from build123d import *

# Parameters (mm, degrees)
EXTRUDE_1_DEPTH = 7.5


with BuildPart() as part:
    # 草图1 → 凸台-拉伸1 (new body, symmetric)
    with BuildSketch(Plane.XY):
        Polygon((1.356773133, 2.35), (-1.356773133, 2.35), (-2.713546265, 0), (-1.356773133, -2.35), (1.356773133, -2.35), (2.713546265, 0), align=None)
    extrude(amount=EXTRUDE_1_DEPTH, both=True)

    # 草图3 → Hole Wizard 387 (revolve, cut)
    with BuildSketch(Plane(origin=(0, 0, 7.5), x_dir=(0, -1, 0), z_dir=(1, 0, 0))):
        Polygon((0, 0), (0, 8.751075774), (1.25, 8), (1.25, 0), align=None)
    hole_wizard_387 = revolve(axis=Axis((0, 0, 13.85), (0, 0, -1)), mode=Mode.SUBTRACT)

    # 镜向1: Hole Wizard 387 across plane
    add(hole_wizard_387.mirror(Plane.XY), mode=Mode.SUBTRACT)


solid = part.part
Design review of the part built by this model. Coordinates are the model's own, in mm. Coordinates: 2 decimals unless noted, no trailing zeros. Write each loop counter-clockwise with the first axis right and the second up, starting at its lowest first coordinate (ties: lowest second). Pieces come first, ordered by that corner, then holes. Notation, with made-up numbers: (40, 85) - (65, 85) arc R12 cw to (65, 99) - close; hole circle Ø4 at (34, 48). An arc over 180 degrees is marked (long way). Use one line per item in the form item = value.
Q1. For probe 1 along Y at (x, z) = (0, -2.25); probe 2 along X at (y, z) = (-1, 5.5); probe 3 along X at (y, z) = (0.5, -4.25), list the stretches that pass through material, from the lowest coordinate up.
Taken from the geometry:
probe_1 = -2.35 to -1.25, 1.25 to 2.35
probe_2 = -2.14 to -0.75, 0.75 to 2.14
probe_3 = -2.42 to -1.15, 1.15 to 2.42
Q2. Consider section D-D (y = 2). Write out the cut boundary in (x, z).
Taken from the geometry:
outline = (-1.56, -7.5) - (1.56, -7.5) - (1.56, 7.5) - (-1.56, 7.5) - close
Q3. Consider section C-C (y = 0.9). Write out the cut boundary in (x, z), plus the area to 3 significant figures.
Taken from the geometry:
outline = (-2.19, -7.5) - (-0.87, -7.5) - (-0.87, 7.5) - (-2.19, 7.5) - close; (0.87, -7.5) - (2.19, -7.5) - (2.19, 7.5) - (0.87, 7.5) - close
area = 39.8 mm^2
Q4. Consider section A-A (x = 0). Write out the cut boundary in (y, z), plus the area to 3 significant figures.
Taken from the geometry:
outline = (-2.35, -7.5) - (-1.25, -7.5) - (-1.25, 7.5) - (-2.35, 7.5) - close; (1.25, -7.5) - (2.35, -7.5) - (2.35, 7.5) - (1.25, 7.5) - close
area = 33.0 mm^2
Q5. The part is to be moulded in two halves that separate along Y. For faces 1 (the flat face through (1, 1, 7.5)), 2 (the cylindrical face through (1.22, 0.27, -0.11)), 3 (the flat face through (-2.045, -1.159, 0.105)), 4 (the flat face through (0, 2.35, 0)), say which applies: +Y half, -Y half, draft (parallel to the pull), parting line (faces both ways), or undercut.
Taken from the geometry:
face_1 = draft
face_2 = undercut
face_3 = -Y half
face_4 = +Y half
Q6. Consider section B-B (z = 4.5). Write out the cut boundary in (x, y), plus the area to 3 significant figures.
Taken from the geometry:
outline = (-2.71, 0) - (-1.36, -2.35) - (1.36, -2.35) - (2.71, 0) - (1.36, 2.35) - (-1.36, 2.35) - close; hole circle Ø2.5 at (0, 0)
area = 14.2 mm^2
